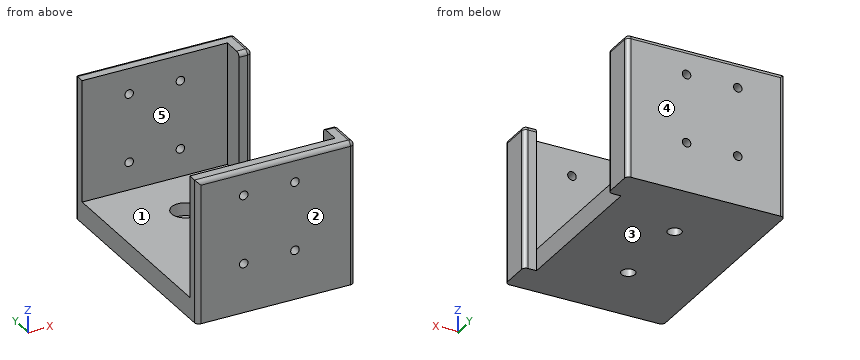
Autodesk Fusion 360 part; units mm, degrees
sketch "Sketch1" plane through (0, 0, 0) normal (0, 0, 1) x (1, 0, 0)
  line L0 (0, 0) -> (34, 0)
  line L1 (34, 0) -> (34, 46.5)
  line L2 (34, 46.5) -> (0, 46.5)
  line L3 (0, 46.5) -> (0, 0)
  dimension "d1" = 34
  dimension "d2" = 46.5
extrude "Extrude1" add sketch "Sketch1" along normal blind 5
sketch "Sketch3" plane through (0, 0, 5) normal (0, 0, 1) x (-1, 0, 0)
  line L0 (-34, 0) -> (-34, -46.5)
  line L1 (-17, 0) -> (-17, -46.5)
  circle A0 centre (-17, -13.25) radius 1.6
  circle A1 centre (-17, -33.25) radius 1.6
  line L2 (0, -46.5) -> (0, 0)
  line L3 (0, 0) -> (-34, 0)
  line L4 (-34, -46.5) -> (0, -46.5)
  dimension "d11" = 3.2
  dimension "d12" = 3.2
  dimension "d13" = 20
hole "Hole1" at (17, 13.25, 5) at (17, 33.25, 5) direction (0, 0, -1) diameter 3.2 depth 5 tip angle 180 counterbore diameter 6.5 counterbore depth 3
sketch "Sketch4" plane through (0, 0, 0) normal (0, 0, -1) x (1, 0, 0)
  circle A0 centre (17, -13.25) radius 1.6
  circle A1 centre (17, -33.25) radius 1.6
  line L0 (0, 0) -> (0, -46.5)
  line L1 (0, -46.5) -> (34, -46.5)
  line L2 (34, -46.5) -> (34, 0)
  line L3 (34, 0) -> (0, 0)
  line L4 (0, -46.5) -> (37, -46.5)
  line L5 (37, -46.5) -> (37, -49.5)
  line L6 (37, -49.5) -> (0, -49.5)
  line L7 (0, -49.5) -> (0, -46.5)
  line L8 (0, 0) -> (37, 0)
  line L9 (37, 0) -> (37, 3)
  line L10 (37, 3) -> (0, 3)
  line L11 (0, 3) -> (0, 0)
  line L12 (37, 0) -> (34, 0)
  line L13 (34, 0) -> (34, -5)
  line L14 (34, -5) -> (37, -5)
  line L15 (37, -5) -> (37, 0)
  line L16 (37, -46.5) -> (34, -46.5)
  line L17 (34, -46.5) -> (34, -41.5)
  line L18 (34, -41.5) -> (37, -41.5)
  line L19 (37, -41.5) -> (37, -46.5)
  dimension "d24" = 37
  dimension "d25" = 3
  dimension "d26" = 37
  dimension "d27" = 3
  dimension "d28" = 5
  dimension "d29" = 5
extrude "Extrude3" add sketch "Sketch4" against normal blind 33.5 contours L3 L8 L9 L10 L11 L12 | L1 L4 L5 L6 L7 L16 | L2 L8 L12 L13 L14 L15 | L2 L4 L16 L17 L18 L19
sketch "Sketch5" plane through (0, -3, 0) normal (0, -1, 0) x (1, 0, 0)
  line L0 (0, 0) -> (37, 0)
  line L1 (37, 0) -> (37, 33.5)
  line L2 (37, 33.5) -> (0, 33.5)
  line L3 (0, 33.5) -> (0, 0)
  circle A0 centre (11, 27.5) radius 1
  circle A1 centre (23, 27.5) radius 1
  circle A2 centre (11, 11.5) radius 1
  circle A3 centre (23, 11.5) radius 1
  dimension "d32" = 2
  dimension "d33" = 6
  dimension "d34" = 11
  dimension "d37" = 12
  dimension "d38" = -16
extrude "Extrude4" cut sketch "Sketch5" against normal blind 52.5 contours A0 | A1 | A2 | A3
fillet "Fillet3" radius 1 12 edges at (35.5, 5, 33.5) (37, 1, 33.5) (18.5, -3, 33.5) (37, -3, 16.75) (37, 5, 16.75) (0, -3, 16.75) (37, 41.5, 16.75) (37, 45.5, 33.5) (35.5, 41.5, 33.5) (37, 49.5, 16.75) (18.5, 49.5, 33.5) (0, 49.5, 16.75)
Design review of the part built by this model. Coordinates are the model's own, in mm. Face numbers are marked on the shaded views. A direction names the side the tool comes from. Coordinates: 2 decimals unless noted, no trailing zeros. Loops run counter-clockwise (first coordinate to the right, second up) from the corner with the lowest first, then second, coordinate; pieces in that order, holes last. Notation, with made-up numbers: (67.5, -21.75) -> (122.5, -21.75) arc R26 cw to (122.5, 6.25) -> close; hole circle Ø8 at (56, -35.5). An arc over 180 degrees is marked (long way). Answer as a JSON object with one key per item and string values.
Q1. Take a section at A-A on z = 17.5. Give the boundary of the cut face in (x, y).
Answer block:
{"outline": "(0, -2) arc R1 ccw to (1, -3) -> (36, -3) arc R1 ccw to (37, -2) -> (37, 4) arc R1 ccw to (36, 5) -> (34, 5) -> (34, 0) -> (0, 0) -> close; (0, 46.5) -> (34, 46.5) -> (34, 41.5) -> (36, 41.5) arc R1 ccw to (37, 42.5) -> (37, 48.5) arc R1 ccw to (36, 49.5) -> (1, 49.5) arc R1 ccw to (0, 48.5) -> close"}
Q2. To check wall thickness, follow L1, parallel to Z at x = 23, y = -1; L2, parallel to Y at x = 17, z = 1.5; L3, parallel to Y at x = 7, z = 20. State the ranges of each line that lie inside material, in increasing order.
Answer block:
{"L1": "z = 0 to 10.5, 12.5 to 26.5, 28.5 to 33.5", "L2": "y = -3 to 11.65, 14.85 to 31.65, 34.85 to 49.5", "L3": "y = -3 to 0, 46.5 to 49.5"}
Q3. Clearance check with flat-ended pins moving along their axes: pin 1 Ø6 at (y, z) = (43, 24.5) entering from -X; pin 2 Ø5 at (x, y) = (17, 33.25) entering from +Z; pin 3 Ø1.8 at (x, z) = (11, 27.5) entering from -Y; pin 4 Ø10 at (x, y) = (17, 32) entering from +Z. State where each tip first meets the part, or that it passes through.
Answer block:
{"pin 1": "stops at x = 34", "pin 2": "stops at z = 2", "pin 3": "passes through", "pin 4": "stops at z = 5"}
Q4. Take a section at B-B on x = 23. Give the boundary of the cut face in (y, z), plus the area to 3 significant figures.
Answer block:
{"outline": "(-3, 0) -> (49.5, 0) -> (49.5, 10.5) -> (46.5, 10.5) -> (46.5, 5) -> (0, 5) -> (0, 10.5) -> (-3, 10.5) -> close; (-3, 12.5) -> (0, 12.5) -> (0, 26.5) -> (-3, 26.5) -> close; (-3, 28.5) -> (0, 28.5) -> (0, 33.5) -> (-2, 33.5) arc R1 ccw to (-3, 32.5) -> close; (46.5, 12.5) -> (49.5, 12.5) -> (49.5, 26.5) -> (46.5, 26.5) -> close; (46.5, 28.5) -> (49.5, 28.5) -> (49.5, 32.5) arc R1 ccw to (48.5, 33.5) -> (46.5, 33.5) -> close", "area": "409 mm^2"}
Q5. The part is to be moulded in two halves that separate along Y. For the marked faces 1, 2 and 3, say which applies: +Y half, -Y half, draft (parallel to the pull), parting line (faces both ways), or undercut.
Answer block:
{"face 1": "undercut", "face 2": "-Y half", "face 3": "draft"}
Q6. Take a section at D-D on z = 11.5. Give the number of separate pieces and of enclosed holes in the cut face, plus the area to 3 significant figures.
Answer block:
{"separate pieces": "6", "enclosed holes": "0", "area": "227 mm^2"}
Q7. Take a section at C-C on y = 13.25. Give the boundary of the cut face in (x, z).
Answer block:
{"outline": "(0, 0) -> (15.4, 0) -> (15.4, 2) -> (13.75, 2) -> (13.75, 5) -> (0, 5) -> close; (18.6, 0) -> (34, 0) -> (34, 5) -> (20.25, 5) -> (20.25, 2) -> (18.6, 2) -> close"}
Q8. Tool access review of the marked faces 4 and 5: name each direction out of +Z, -Z, +X, -X, +Y, -Y from which nothing blocks a thin tool from reaching the whole face with its end or side.
Answer block:
{"face 4": "+Z, -Z, +X, -X, +Y", "face 5": "+Z, -X"}
